```python
from build123d import *

# Parameters (mm, degrees)
SKETCH1_W           = 10
SKETCH1_H           = 5.3
BOSS_EXTRUDE1_DEPTH = 7
SKETCH3_W           = 8.8
SKETCH3_H           = 4
CUT_EXTRUDE1_DEPTH  = 5
SKETCH4_W           = 1.2
SKETCH4_H           = 5
CUT_EXTRUDE2_DEPTH  = 4
SKETCH5_W           = 10
SKETCH5_H           = 0.8
CUT_EXTRUDE3_DEPTH  = 0.8
SKETCH6_W           = 0.8
SKETCH6_H           = 0.8
CUT_EXTRUDE4_DEPTH  = 10
SKETCH7_W           = 8.8
SKETCH7_H           = 1
CUT_EXTRUDE5_DEPTH  = 0.3


with BuildPart() as part:
    # Sketch1 → Boss-Extrude1 (new body)
    with BuildSketch(Plane(origin=(0, 0, 0), x_dir=(1, 0, 0), z_dir=(0, 1, 0))):
        Rectangle(SKETCH1_W, SKETCH1_H)
    extrude(amount=BOSS_EXTRUDE1_DEPTH)

    # Sketch3 → Cut-Extrude1 (cut)
    with BuildSketch(Plane.XZ):
        Rectangle(SKETCH3_W, SKETCH3_H)
    extrude(amount=-CUT_EXTRUDE1_DEPTH, mode=Mode.SUBTRACT)

    # Sketch4 → Cut-Extrude2 (cut)
    with BuildSketch(Plane.XY.offset(2.65)):
        with Locations((-3.4, 2.5)):
            Rectangle(SKETCH4_W, SKETCH4_H)
        with Locations((3.4, 2.5)):
            Rectangle(SKETCH4_W, SKETCH4_H)
    extrude(amount=-CUT_EXTRUDE2_DEPTH, mode=Mode.SUBTRACT)

    # Sketch5 → Cut-Extrude3 (cut)
    with BuildSketch(Plane(origin=(0, 7, 0), x_dir=(1, 0, 0), z_dir=(0, 1, 0))):
        with Locations((0, 2.25)):
            Rectangle(SKETCH5_W, SKETCH5_H)
    extrude(amount=-CUT_EXTRUDE3_DEPTH, mode=Mode.SUBTRACT)

    # Sketch6 → Cut-Extrude4 (cut)
    with BuildSketch(Plane(origin=(0, 7, 0), x_dir=(1, 0, 0), z_dir=(0, 1, 0))):
        with Locations((2.55, -0.65)):
            Rectangle(SKETCH6_W, SKETCH6_H)
        with Locations((-0.15, -0.65)):
            Rectangle(SKETCH6_W, SKETCH6_H)
        with Locations((-2.75, -0.65)):
            Rectangle(SKETCH6_W, SKETCH6_H)
    extrude(amount=-CUT_EXTRUDE4_DEPTH, mode=Mode.SUBTRACT)

    # Sketch7 → Cut-Extrude5 (cut)
    with BuildSketch(Plane.XZ.offset(-5)):
        with Locations((0, -1.5)):
            Rectangle(SKETCH7_W, SKETCH7_H)
    extrude(amount=-CUT_EXTRUDE5_DEPTH, mode=Mode.SUBTRACT)


solid = part.part
```
Source: CAD feature listing. Evaluate the final solid. Frame: model axes, mm. A direction names the side the tool comes from. Give positions to 0.01 mm unless a question says otherwise; leave off trailing zeros. Write each loop counter-clockwise with the first axis right and the second up, starting at its lowest first coordinate (ties: lowest second). Pieces come first, ordered by that corner, then holes. Notation, with made-up numbers: (62, 72.5) - (93, 72.5) arc R36 ccw to (93, 107.5) - close; hole circle Ø7 at (-5.75, 43). An arc over 180 degrees is marked (long way). One line per item, written item: value. Start each with the question number.
Q1. Material intervals for probe 1 along X at (y, z) = (2.5, 2.3); probe 2 along Z at (x, y) = (-2.75, 3); probe 3 along X at (y, z) = (3, 0.1), sorted ascending. Write a range as from..to.
Q2. First-contact query: pin 1 Ø0.8 at (x, z) = (1, -1.5) entering from -Y. Flat tip, straight axial feed; report the tip coordinate or a pass-through.
Q3. Set-up query: faces 5 (the face through (0, 3, 2.65)), 6 (the face through (0, 3, -2)), 7 (the face through (2.5, 6, 1.05)). Return all of +Z, -Z, +X, -X, +Y, -Y with unobstructed straight access to the full face (end or side cutting, diameter ignored); none if empty.
Q4. Section query A-A, the plane x = 0. Return the cut outline in (y, z).
Q5. Section query B-B, the plane z = 0.6. Return the cut outline in (x, y).
Q6. Draft query along X for faces 1 (the face through (-4.4, 3, 0)), 2 (the face through (0, 7, 0)), 3 (the face through (-5, 3, 0)), 4 (the face through (2.5, 6, 0.25)). Return one class per face: +X half, -X half, draft (parallel to the pull), parting line (faces both ways), or undercut.
Q7. Section query D-D, the plane x = -1.75. Return the cut outline in (y, z).
Q8. Section query C-C, the plane y = 3.25. Return the cut outline in (x, z), then the cut area to 3 significant figures.
Answer:
1. probe 1: x = -5..-4, -2.8..2.8, 4..5
1. probe 2: z = -2.65..-2, 2..2.65
1. probe 3: x = -5..-4.4, 4.4..5
2. pin 1: stops at y = 5.3
3. face 5: +Z, +X, -X, +Y, -Y
3. face 6: -Y
3. face 7: +Y, -Y
4. outline: (0, -2.65) - (6.2, -2.65) - (6.2, -1.85) - (7, -1.85) - (7, 0.25) - (5, 0.25) - (5, -1) - (5.3, -1) - (5.3, -2) - (0, -2) - close; (0, 2) - (5, 2) - (5, 1.05) - (7, 1.05) - (7, 2.65) - (0, 2.65) - close
5. outline: (-5, 0) - (-4.4, 0) - (-4.4, 5) - (-3.15, 5) - (-3.15, 7) - (-5, 7) - close; (-2.35, 5) - (-0.55, 5) - (-0.55, 7) - (-2.35, 7) - close; (0.25, 5) - (2.15, 5) - (2.15, 7) - (0.25, 7) - close; (2.95, 5) - (4.4, 5) - (4.4, 0) - (5, 0) - (5, 7) - (2.95, 7) - close
6. face 1: undercut
6. face 2: draft
6. face 3: -X half
6. face 4: undercut
7. outline: (0, -2.65) - (6.2, -2.65) - (6.2, -1.85) - (7, -1.85) - (7, 2.65) - (0, 2.65) - (0, 2) - (5, 2) - (5, -1) - (5.3, -1) - (5.3, -2) - (0, -2) - close
8. outline: (-5, -2.65) - (5, -2.65) - (5, 2.65) - (4, 2.65) - (4, 2) - (4.4, 2) - (4.4, -2) - (-4.4, -2) - (-4.4, 2) - (-4, 2) - (-4, 2.65) - (-5, 2.65) - close; (-2.8, 2) - (2.8, 2) - (2.8, 2.65) - (-2.8, 2.65) - close
8. area: 16.2 mm2
